```python
from build123d import *

# Parameters (mm, degrees)
F1_DEPTH = 3
F2_R     = 1.5
F3_DEPTH = 3.001


with BuildPart() as f1:
    # F0 (on Top) → F1 (new body)
    with BuildSketch(Plane.XY):
        Polygon((0, 3.175426), (-2.75, 1.587713), (-2.75, -1.587713), (0, -3.175426), (2.75, -1.587713), (2.75, 1.587713), align=None)
    extrude(amount=F1_DEPTH)

    # F2 (on face) → F3 (cut, through all)
    with BuildSketch(Plane.XY.offset(3)):
        Circle(F2_R)
    extrude(amount=-F3_DEPTH, mode=Mode.SUBTRACT)


solid = f1.part
```
Geometry check sheet. Reference: the model listing, model coordinates, mm. Give positions to 0.01 mm unless a question says otherwise; leave off trailing zeros. Write each loop counter-clockwise with the first axis right and the second up, starting at its lowest first coordinate (ties: lowest second). Pieces come first, ordered by that corner, then holes. Notation, with made-up numbers: (-31, 61.5) -> (27, 61.5) arc R16 ccw to (27, 73.5) -> close; hole circle Ø1 at (-2, -26.5). An arc over 180 degrees is marked (long way). One line per question, with ' | ' between items.
Item 1: Sectioned sample at D-D, the plane x = 1.85. Record the boundary of the cut face in (y, z).
Determined:
outline: (-2.11, 0) -> (2.11, 0) -> (2.11, 3) -> (-2.11, 3) -> close
Item 2: Draft check along X on faces 1 (the flat face through (-1.3, -1.4, 3)), 2 (the cylindrical face through (-1.5, 0.07, 1.52)), 3 (the flat face through (-1.36, 2.39, 1.48)), 4 (the flat face through (2.75, 0, 1)). Enter one of: released by +X, released by -X, zero draft, split by the parting line, or undercut.
Determined:
face 1: zero draft | face 2: undercut | face 3: released by -X | face 4: released by +X
Item 3: Sectioned sample at C-C, the plane x = -1.1. Record the boundary of the cut face in (y, z).
Determined:
outline: (-2.54, 0) -> (-1.02, 0) -> (-1.02, 3) -> (-2.54, 3) -> close; (1.02, 0) -> (2.54, 0) -> (2.54, 3) -> (1.02, 3) -> close
Item 4: Sectioned sample at A-A, the plane y = 0. Record the boundary of the cut face in (x, z), plus the area to 3 significant figures.
Determined:
outline: (-2.75, 0) -> (-1.5, 0) -> (-1.5, 3) -> (-2.75, 3) -> close; (1.5, 0) -> (2.75, 0) -> (2.75, 3) -> (1.5, 3) -> close | area: 7.50 mm^2
Item 5: Sectioned sample at B-B, the plane z = 2.2. Record the boundary of the cut face in (x, y).
Determined:
outline: (-2.75, -1.59) -> (0, -3.18) -> (2.75, -1.59) -> (2.75, 1.59) -> (0, 3.18) -> (-2.75, 1.59) -> close; hole circle Ø3 at (0, 0)
Item 6: Depth check by flat-ended pin: pin 1 (1 mm diameter, centred on x = -2, z = 2, fed in from -Y). Enter the tip coordinate at first touch or a pass-through.
Determined:
pin 1: y = -2.31
Item 7: Scan lines: line 1 along Y through (x, z) = (-0.2, 1.4); line 2 along Y through (x, z) = (-0.5, 1.95); line 3 along X through (y, z) = (0.5, 2.45). Record each from-to range of solid material in increasing order.
Determined:
line 1: -3.06 to -1.49, 1.49 to 3.06 | line 2: -2.89 to -1.41, 1.41 to 2.89 | line 3: -2.75 to -1.41, 1.41 to 2.75
